```python
from build123d import *

# Parameters (mm, degrees)
PAD_DEPTH       = 20
SKETCH001_R     = 2.55
POCKET_DEPTH    = 22.0443961318
SKETCH002_R     = 2.55
POCKET001_DEPTH = 10
SKETCH003_R     = 5
POCKET002_DEPTH = 3.5
POCKET003_DEPTH = 16.2
FILLET_R        = 1


with BuildPart() as part:
    # Sketch → Pad (new body)
    with BuildSketch(Plane.XY):
        Polygon((-35, 0), (-35, 9), (-19.949111567, 9), (-19.949111567, 16), (-17.8645079021, 22.0433961318), (19.949111567, 9), (35, 9), (35, 0), align=None)
    extrude(amount=PAD_DEPTH)

    # Sketch001 (on Face8 of Pad) → Pocket (cut, through all)
    with BuildSketch(Plane.XZ):
        with Locations((-27, 10)):
            Circle(SKETCH001_R)
        with Locations((27, 10)):
            Circle(SKETCH001_R)
    extrude(amount=-POCKET_DEPTH, mode=Mode.SUBTRACT)

    # Sketch002 (on Face11 of Pocket) → Pocket001 (cut)
    with BuildSketch(Plane(origin=(4.8955675974, 14.1925560139, 0), x_dir=(-0.9453404867, 0.3260849033, 0), z_dir=(0.3260849033, 0.9453404867, 0))):
        with Locations((-5.9239387088, 10)):
            Circle(SKETCH002_R)
        with Locations((14.0760612912, 10)):
            Circle(SKETCH002_R)
    extrude(amount=-POCKET001_DEPTH, mode=Mode.SUBTRACT)

    # Sketch003 (on Face12 of Pocket001) → Pocket002 (cut)
    with BuildSketch(Plane(origin=(0, 9, 0), x_dir=(-1, 0, 0), z_dir=(0, 1, 0))):
        with Locations((-27, 10)):
            Circle(SKETCH003_R)
        with Locations((27, 10)):
            Circle(SKETCH003_R)
    extrude(amount=-POCKET002_DEPTH, mode=Mode.SUBTRACT)

    # Sketch004 (on Face4 of Pocket002) → Pocket003 (cut)
    with BuildSketch(Plane(origin=(0, 0, 0), x_dir=(1, 0, 0), z_dir=(0, 0, -1))):
        Polygon((-14.9184124801, -13.4108691689), (-6.5994161969, -10.5413220199), (-5.2298596031, -14.5117520642), (-13.5488558863, -17.3812992131), align=None)
        Polygon((3.9883972544, -6.889171103), (5.3579538482, -10.8596011473), (13.6769501314, -7.9900539983), (12.3073935376, -4.019623954), align=None)
    extrude(amount=-POCKET003_DEPTH, mode=Mode.SUBTRACT)

    # Fillet
    fillet_edges = [part.edges().sort_by_distance(p)[0] for p in [
        (0, 0, 0),
        (-35, 0, 10),
        (-35, 4.5, 0),
        (-35, 9, 10),
        (-27.474556, 9, 0),
        (1.042302, 15.521698, 0),
        (27.474556, 9, 0),
        (35, 4.5, 0),
        (-18.90681, 19.021698, 0),
        (-19.949112, 16, 10),
        (-19.949112, 12.5, 0),
        (35, 9, 10),
        (-17.864508, 22.043396, 10),
        (-18.90681, 19.021698, 20),
        (-19.949112, 12.5, 20),
        (-27.474556, 9, 20),
        (0, 0, 20),
        (27.474556, 9, 20),
        (35, 4.5, 20),
        (1.042302, 15.521698, 20),
        (19.949112, 9, 10),
        (-19.949112, 9, 10),
        (32, 9, 10),
        (-22, 9, 10),
    ]]
    fillet(fillet_edges, radius=FILLET_R)


solid = part.part
```
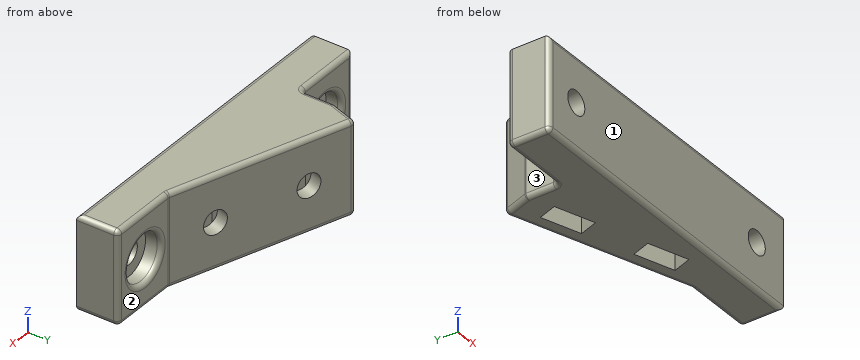
For this review, take the finished solid that the model builds, in its own axes (mm). Face numbers are marked on the shaded views. A direction names the side the tool comes from. Round coordinates to 2 decimals unless told otherwise and drop trailing zeros. Write each loop counter-clockwise with the first axis right and the second up, starting at its lowest first coordinate (ties: lowest second). Pieces come first, ordered by that corner, then holes. Notation, with made-up numbers: (-19.75, 49.25) - (0.25, 49.25) arc R5 ccw to (0.25, 58.25) - close; hole circle Ø9 at (53.5, 17). An arc over 180 degrees is marked (long way). Answer as a JSON object with one key per item and string values.
1. We need section C-C on z = 10. Count the separate pieces of the cut face and the enclosed holes in it, then the cut area to 3 significant figures.
Response values:
{"separate pieces": "3", "enclosed holes": "0", "area": "637 mm2"}
2. For pin 1 Ø5.5 at (x, y) = (-9, 15.5) entering from -Z; pin 2 Ø6.5 at (x, z) = (-29, 13) entering from +Y; pin 3 Ø2 at (y, z) = (19.5, 14) entering from -X; pin 4 Ø5 at (x, z) = (17.5, 3) entering from +Y, all flat-tipped, find the tip position at first contact; note any pin that passes through.
Response values:
{"pin 1": "stops at z = 0", "pin 2": "stops at y = 9", "pin 3": "stops at x = -19.09", "pin 4": "stops at y = 10.71"}
3. We need section B-B on z = 17.25. Give the boundary of the cut face in (x, y), then the cut area to 3 significant figures.
Response values:
{"outline": "(-35, 1) arc R1 ccw to (-34, 0) - (35, 0) - (35, 8) arc R1 ccw to (34, 9) - (20.12, 9) arc R1 cw to (19.79, 9.05) - (-16.92, 21.72) arc R1 ccw to (-18.19, 21.1) - (-19.89, 16.16) arc R1 ccw to (-19.95, 15.83) - (-19.95, 10) arc R1 cw to (-20.95, 9) - (-34, 9) arc R1 ccw to (-35, 8) - close", "area": "897 mm2"}
4. We need section A-A on x = -27. Give the boundary of the cut face in (y, z).
Response values:
{"outline": "(0, 1) arc R1 ccw to (1, 0) - (8, 0) arc R1 ccw to (9, 1) - (9, 4) arc R1 ccw to (8, 5) - (5.5, 5) - (5.5, 7.45) - (0, 7.45) - close; (0, 12.55) - (5.5, 12.55) - (5.5, 15) - (8, 15) arc R1 ccw to (9, 16) - (9, 19) arc R1 ccw to (8, 20) - (1, 20) arc R1 ccw to (0, 19) - close"}
5. Tool access review of the marked faces 1, 2 and 3: name each direction out of +Z, -Z, +X, -X, +Y, -Y from which nothing blocks a thin tool from reaching the whole face with its end or side.
Response values:
{"face 1": "+Z, -Z, +X, -X, -Y", "face 2": "+Z, -Z, +X, +Y", "face 3": "+Z, -Z, -X, +Y"}
6. To check wall thickness, follow line 1 along Z through (x, y) = (27, 6.1); line 2 along Z through (x, y) = (27, 3.25); line 3 along Z through (x, y) = (-10, 16). State the ranges of each line that lie inside material, in increasing order.
Response values:
{"line 1": "z = 0 to 5, 15 to 20", "line 2": "z = 0 to 7.45, 12.55 to 20", "line 3": "z = 16.2 to 20"}
